Input: part model. Units: mm. Frame: model coordinates. Round coordinates to 2 decimals unless told otherwise and drop trailing zeros. Loops run counter-clockwise (first coordinate to the right, second up) from the corner with the lowest first, then second, coordinate; pieces in that order, holes last. Notation, with made-up numbers: (-5.5, 9) -> (22.5, 9) arc R12 ccw to (22.5, 24) -> close; hole circle Ø10 at (22.25, 26). An arc over 180 degrees is marked (long way). One line per question, with ' | ' between items. Start each with the question number.
Q1. Cut plane A-A on y = 47. Return loops of the section in (x, z), and give its area (3 significant figures).
Q2. Contact query for flat-ended pins moving along their axis: P1, Ø1, axis at x = -25.5, z = 1.5, coming from the -Y side; P2, Ø1, axis at y = -22.5, z = 3.5, coming from the -X side; P3, Ø4, axis at x = -29.5, y = 27.5, coming from the +Z side. Output: stop coordinate, or through.
Q3. Cut plane C-C on x = -34.25. State how many separate pieces and enclosed holes the cut face has, and give its area (3 significant figures).
Q4. Cut plane B-B on z = 3.65. Return loops of the section in (x, y), and give its area (3 significant figures).
Q5. Material intervals for L1, parallel to X at y = 21.5, z = 1.1; L2, parallel to X at y = -20.5, z = 1.7; L3, parallel to X at y = 7.5, z = 2.55, sorted ascending.
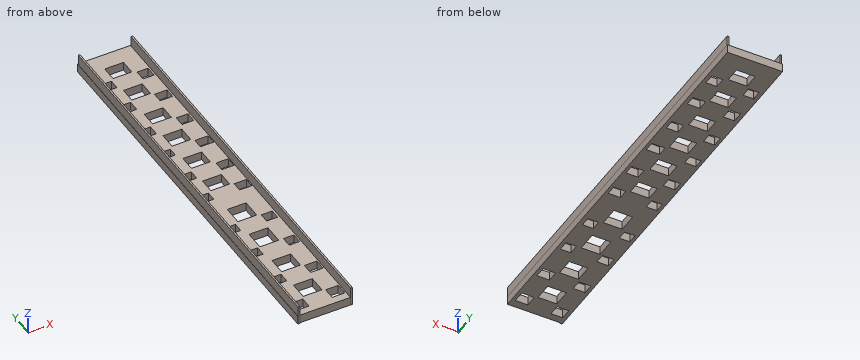
from build123d import *

# Parameters (mm, degrees)
F0_W     = 13.074241
F0_H     = 94.193969
F0_W_2   = 2.772734
F0_H_2   = 2.638768
F0_W_3   = 2.816748
F0_H_3   = 2.462851
F0_W_4   = 2.767764
F0_H_4   = 2.35983
F0_W_5   = 4.457127
F0_H_5   = 4.159985
F0_H_6   = 4.159987
F0_W_6   = 2.510216
F0_H_7   = 2.259195
F0_W_7   = 2.54634
F0_H_8   = 2.325126
F0_H_9   = 4.663303
F0_H_10  = 4.562473
F0_H_11  = 3.565702
F0_W_8   = 2.992794
F0_H_12  = 2.814685
F0_W_9   = 2.481149
F0_H_13  = 2.474324
F0_W_10  = 2.581937
F0_H_14  = 2.295056
F0_W_11  = 2.870289
F0_W_12  = 2.812862
F0_H_15  = 2.324136
F0_W_13  = 2.721176
F0_H_16  = 2.166863
F0_W_14  = 2.620392
F0_H_17  = 2.519607
F0_H_18  = 3.660711
F0_H_19  = 3.862843
F0_W_15  = 2.633039
F0_H_20  = 2.633039
F0_W_16  = 2.51843
F0_H_21  = 2.364244
F0_H_22  = 3.565703
F0_W_17  = 2.904148
F0_H_23  = 2.471199
F0_W_18  = 3.174707
F0_H_24  = 2.368433
F0_W_19  = 2.771571
F0_H_25  = 2.469215
F0_W_20  = 2.967037
F0_H_26  = 2.430499
F0_W_21  = 2.61249
F0_H_27  = 2.569832
F1_DEPTH = 2.032
F2_W     = 0.389233
F2_H     = 94.105582
F2_W_2   = 0.415065
F2_H_2   = 94.00139
F3_DEPTH = 4.572


with BuildPart() as f1:
    # F0 (on Top) → F1 (new body)
    with BuildSketch(Plane.XY):
        with Locations((-29.882617, 9.551766)):
            Rectangle(F0_W, F0_H)
        with Locations((-34.133058, -34.544973)):
            Rectangle(F0_W_2, F0_H_2, mode=Mode.SUBTRACT)
        with Locations((-34.199076, -25.177347)):
            Rectangle(F0_W_3, F0_H_3, mode=Mode.SUBTRACT)
        with Locations((-34.223568, -15.219573)):
            Rectangle(F0_W_4, F0_H_4, mode=Mode.SUBTRACT)
        with Locations((-30.031188, -30.413814)):
            Rectangle(F0_W_5, F0_H_5, mode=Mode.SUBTRACT)
        with Locations((-30.031188, -21.202417)):
            Rectangle(F0_W_5, F0_H_6, mode=Mode.SUBTRACT)
        with Locations((-34.39744, -6.244165)):
            Rectangle(F0_W_6, F0_H_7, mode=Mode.SUBTRACT)
        with Locations((-34.379378, 5.415873)):
            Rectangle(F0_W_7, F0_H_8, mode=Mode.SUBTRACT)
        with Locations((-30.031188, -11.648393)):
            Rectangle(F0_W_5, F0_H_9, mode=Mode.SUBTRACT)
        with Locations((-30.031188, -2.281236)):
            Rectangle(F0_W_5, F0_H_10, mode=Mode.SUBTRACT)
        with Locations((-30.031188, 8.808911)):
            Rectangle(F0_W_5, F0_H_11, mode=Mode.SUBTRACT)
        with Locations((-25.660809, -34.281095)):
            Rectangle(F0_W_8, F0_H_12, mode=Mode.SUBTRACT)
        with Locations((-25.660809, -25.089389)):
            Rectangle(F0_W_8, F0_H_2, mode=Mode.SUBTRACT)
        with Locations((-25.457825, -15.217207)):
            Rectangle(F0_W_9, F0_H_13, mode=Mode.SUBTRACT)
        with Locations((-25.647538, -6.118654)):
            Rectangle(F0_W_10, F0_H_14, mode=Mode.SUBTRACT)
        with Locations((-25.503362, 5.490877)):
            Rectangle(F0_W_11, F0_H_8, mode=Mode.SUBTRACT)
        with Locations((-34.246117, 13.206795)):
            Rectangle(F0_W_12, F0_H_15, mode=Mode.SUBTRACT)
        with Locations((-34.430865, 21.862716)):
            Rectangle(F0_W_13, F0_H_16, mode=Mode.SUBTRACT)
        with Locations((-34.430865, 30.051447)):
            Rectangle(F0_W_14, F0_H_17, mode=Mode.SUBTRACT)
        with Locations((-30.031188, 17.188502)):
            Rectangle(F0_W_5, F0_H_18, mode=Mode.SUBTRACT)
        with Locations((-30.031188, 25.597425)):
            Rectangle(F0_W_5, F0_H_19, mode=Mode.SUBTRACT)
        with Locations((-34.155721, 39.043644)):
            Rectangle(F0_W_15, F0_H_20, mode=Mode.SUBTRACT)
        with Locations((-34.239542, 47.121396)):
            Rectangle(F0_W_16, F0_H_21, mode=Mode.SUBTRACT)
        with Locations((-30.031188, 33.768827)):
            Rectangle(F0_W_5, F0_H_11, mode=Mode.SUBTRACT)
        with Locations((-30.031188, 42.683085)):
            Rectangle(F0_W_5, F0_H_22, mode=Mode.SUBTRACT)
        with Locations((-30.031188, 50.705915)):
            Rectangle(F0_W_5, F0_H_22, mode=Mode.SUBTRACT)
        with Locations((-25.486433, 13.164537)):
            Rectangle(F0_W_17, F0_H_23, mode=Mode.SUBTRACT)
        with Locations((-25.637428, 21.812324)):
            Rectangle(F0_W_18, F0_H_24, mode=Mode.SUBTRACT)
        with Locations((-25.637428, 30.076643)):
            Rectangle(F0_W_19, F0_H_25, mode=Mode.SUBTRACT)
        with Locations((-25.73516, 39.043646)):
            Rectangle(F0_W_20, F0_H_26, mode=Mode.SUBTRACT)
        with Locations((-25.557887, 47.07)):
            Rectangle(F0_W_21, F0_H_27, mode=Mode.SUBTRACT)
    extrude(amount=F1_DEPTH)

    # F2 (on Top) → F3 (join)
    with BuildSketch(Plane.XY):
        with Locations((-36.159336, 9.322742)):
            Rectangle(F2_W, F2_H)
        with Locations((-23.633422, 9.399328)):
            Rectangle(F2_W_2, F2_H_2)
    extrude(amount=F3_DEPTH)


solid = f1.part
Results:
1) outline: (-36.42, 0) -> (-35.5, 0) -> (-35.5, 2.03) -> (-35.96, 2.03) -> (-35.96, 4.57) -> (-36.35, 4.57) -> (-36.35, 2.03) -> (-36.42, 2.03) -> close; (-32.98, 0) -> (-26.86, 0) -> (-26.86, 2.03) -> (-32.98, 2.03) -> close; (-24.25, 0) -> (-23.35, 0) -> (-23.35, 2.03) -> (-23.43, 2.03) -> (-23.43, 4.57) -> (-23.84, 4.57) -> (-23.84, 2.03) -> (-24.25, 2.03) -> close | area: 18.2 mm^2
2) P1: y = -37.55 | P2: x = -36.35 | P3: z = 2.03
3) separate pieces: 11 | enclosed holes: 0 | area: 143 mm^2
4) outline: (-36.35, -37.73) -> (-35.96, -37.73) -> (-35.96, 56.38) -> (-36.35, 56.38) -> close; (-23.84, -37.6) -> (-23.43, -37.6) -> (-23.43, 56.4) -> (-23.84, 56.4) -> close | area: 75.6 mm^2
5) L1: -36.42 to -35.79, -33.07 to -27.22, -24.05 to -23.35 | L2: -36.42 to -32.26, -27.8 to -23.35 | L3: -36.35 to -35.96, -23.84 to -23.43
